from build123d import *

# Parameters (mm, degrees)
SKETCH1_W           = 9.5
SKETCH1_H           = 8.5
BOARD_OUTLINE_DEPTH = 1.6
SKETCH2_R           = 0.6
SKETCH2_R_2         = 1.6
SKETCH2_R_3         = 0.127
NPTH_DEPTH          = 13.49739973


with BuildPart() as part:
    # Sketch1 → Board_Outline (new body)
    with BuildSketch(Plane.XY):
        with Locations((4.5, 4)):
            Rectangle(SKETCH1_W, SKETCH1_H)
    extrude(amount=BOARD_OUTLINE_DEPTH)

    # Sketch2 → NPTH (cut, through all)
    with BuildSketch(Plane.XY):
        with Locations((8, 7)):
            Circle(SKETCH2_R)
        with Locations((1, 7)):
            Circle(SKETCH2_R)
        with Locations((1, 1)):
            Circle(SKETCH2_R)
        with Locations((8, 1)):
            Circle(SKETCH2_R)
        with Locations((4.5, 4)):
            Circle(SKETCH2_R_2)
        with Locations((2.7, 2.3)):
            Circle(SKETCH2_R_3)
        with Locations((6.2, 1.4)):
            Circle(SKETCH2_R_3)
        with Locations((2.9, 6.7492)):
            Circle(SKETCH2_R_3)
        with Locations((2.921, 5.842)):
            Circle(SKETCH2_R_3)
        with Locations((6.4516, 2.2352)):
            Circle(SKETCH2_R_3)
        with Locations((6.985, 6.1214)):
            Circle(SKETCH2_R_3)
    extrude(amount=NPTH_DEPTH, mode=Mode.SUBTRACT)


solid = part.part
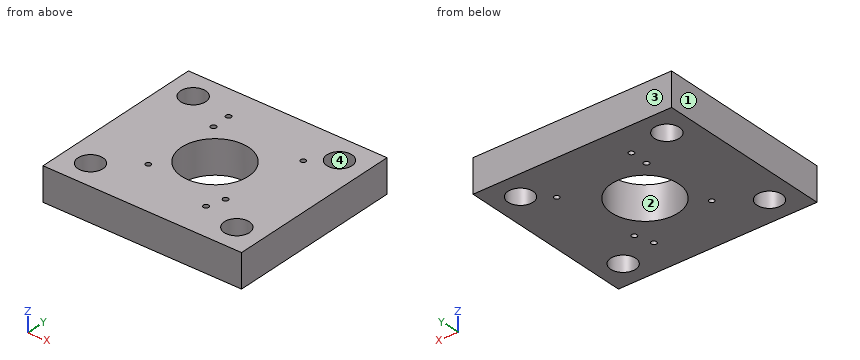
Source: CAD feature listing. Evaluate the final solid. Frame: model axes, mm. Face numbers are marked on the shaded views. Round coordinates to 2 decimals unless told otherwise and drop trailing zeros. Write each loop counter-clockwise with the first axis right and the second up, starting at its lowest first coordinate (ties: lowest second). Pieces come first, ordered by that corner, then holes. Notation, with made-up numbers: (-5.5, 56.5) - (44.5, 56.5) arc R22 ccw to (44.5, 83.5) - close; hole circle Ø6 at (76.5, 43.5). An arc over 180 degrees is marked (long way). Use CSV: the item, a comma, the result in double quotes. Start each with the question number.
(1) Mould query, pull axis Y, two halves, no side actions, for the marked faces 1, 2, 3 and 4. Classes: pulls with the +Y half, pulls with the -Y half, needs draft (parallel to the pull), parting line crosses it, or undercut.
(2) Material intervals for probe 1 along Y at (x, z) = (1, 0.45); probe 2 along X at (y, z) = (1, 0.6); probe 3 along X at (y, z) = (7.25, 0.45), sorted ascending. Write a range as [from, to].
(3) Cut plane B-B, the plane y = 1. Return loops of the section in (x, z), and give its area (3 significant figures).
(4) Cut plane D-D, the plane z = 0.7. Give the number of separate pieces and of enclosed holes in the cut face, and give its area (3 significant figures).
(5) Cut plane A-A, the plane x = 4.5. Return loops of the section in (y, z), and give its area (3 significant figures).
(6) Cut plane C-C, the plane x = 1. Return loops of the section in (y, z).
Geometry says:
1,face 1,"needs draft"
1,face 2,"undercut"
1,face 3,"pulls with the +Y half"
1,face 4,"undercut"
2,probe 1,"[-0.25, 0.4], [1.6, 6.4], [7.6, 8.25]"
2,probe 2,"[-0.25, 0.4], [1.6, 7.4], [8.6, 9.25]"
2,probe 3,"[-0.25, 0.45], [1.55, 7.45], [8.55, 9.25]"
3,outline,"(-0.25, 0) - (0.4, 0) - (0.4, 1.6) - (-0.25, 1.6) - close; (1.6, 0) - (7.4, 0) - (7.4, 1.6) - (1.6, 1.6) - close; (8.6, 0) - (9.25, 0) - (9.25, 1.6) - (8.6, 1.6) - close"
3,area,"11.4 mm²"
4,separate pieces,"1"
4,enclosed holes,"11"
4,area,"67.9 mm²"
5,outline,"(-0.25, 0) - (2.4, 0) - (2.4, 1.6) - (-0.25, 1.6) - close; (5.6, 0) - (8.25, 0) - (8.25, 1.6) - (5.6, 1.6) - close"
5,area,"8.48 mm²"
6,outline,"(-0.25, 0) - (0.4, 0) - (0.4, 1.6) - (-0.25, 1.6) - close; (1.6, 0) - (6.4, 0) - (6.4, 1.6) - (1.6, 1.6) - close; (7.6, 0) - (8.25, 0) - (8.25, 1.6) - (7.6, 1.6) - close"
